Design review of the part built by this model. Coordinates are the model's own, in mm. Coordinates: 2 decimals unless noted, no trailing zeros. Loops run counter-clockwise (first coordinate to the right, second up) from the corner with the lowest first, then second, coordinate; pieces in that order, holes last.
Q1. Add section C-C on x = 29. Give the boundary of the cut face in (y, z), and give its area (3 significant figures).
Q2. Wall thickness on probe 1 along Y at (x, z) = (89, 3.15); probe 2 along Y at (x, z) = (94.5, 4.6); probe 3 along Y at (x, z) = (20, 1.6): over which ranges is each line inside the solid? List them lowest first.
Q3. For P1, Ø1.4, axis at y = -38, z = 3.5, coming from the +X side; P2, Ø2, axis at x = 10.5, z = 1.5, coming from the -Y side; P3, Ø3, axis at x = 85, z = 3.5, coming from the +Y side; P4, Ø2, axis at x = 28, y = -12.5, coming from the -Z side, all flat-tipped, find the tip position at first contact; note any pin that passes through.
Q4. Add section B-B on y = -24. Give the boundary of the cut face in (x, z).
Q5. Add section A-A on x = 94. Give the boundary of the cut face in (y, z).
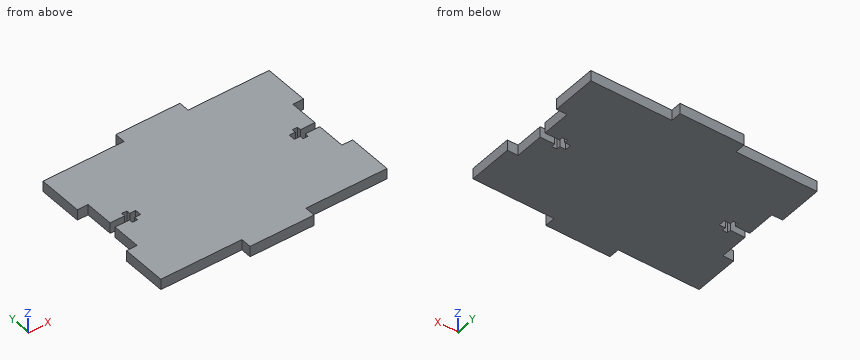
Autodesk Inventor part; units mm, degrees
ref_plane "工作平面2" through (-5, -77, -121) normal (-1, 0, 0) x (0, 0, 1)
ref_plane "工作平面3" through (101, -77, -121) normal (1, 0, 0) x (0, 1, 0)
ref_plane "YZ Plane" through (0, 0, 0) normal (1, 0, 0) x (0, 1, 0)
sketch "slot" plane through (0, 0, 0) normal (0, 0, 1) x (1, 0, 0)
  line L0 (-18.25, 14.2) -> (-11.75, 11.8) construction
  line L1 (-11.75, 14.2) -> (-18.25, 11.8) construction
  line L2 (-18.25, 14.2) -> (-16.5, 14.2)
  line L3 (-13.5, 14.2) -> (-11.75, 14.2)
  line L4 (-16.5, 9) -> (-16.5, 11.8)
  line L5 (-16.5, 14.2) -> (-16.5, 21)
  line L6 (-13.5, 21) -> (-13.5, 14.2)
  line L7 (-13.5, 11.8) -> (-13.5, 9)
  line L8 (-11.75, 11.8) -> (-13.5, 11.8)
  line L9 (-16.5, 11.8) -> (-18.25, 11.8)
  line L10 (-16.5, 21) -> (-13.5, 21)
  line L11 (-13.5, 9) -> (-16.5, 9)
  line L12 (-11.75, 14.2) -> (-11.75, 11.8)
  line L13 (-18.25, 11.8) -> (-18.25, 14.2)
  point P0 (-15, 21)
  point P1 (-15, 13)
  dimension "d8" = 3
  dimension "d9" = 12
  dimension "d10" = 6.5
  dimension "d11" = 2.4
  dimension "d12" = 8
ref_plane "工作平面1" through (0, 0, 0) normal (0, 0, 1) x (1, 0, 0)
sketch "草图2" plane through (0, 0, 0) normal (0, 0, 1) x (1, 0, 0)
  line L0 (74, -10) -> (74, -69)
  line L1 (74, -69) -> (69, -69)
  line L2 (69, -69) -> (69, -10)
  line L3 (69, -10) -> (74, -10)
  circle A0 centre (48, 2.5) radius 1.5
  circle A1 centre (48, -74.5) radius 1.5
  line L4 (33, -77) -> (33, -72)
  line L5 (63, -77) -> (33, -77)
  line L6 (63, -72) -> (63, -77)
  line L7 (96, -72) -> (63, -72)
  line L8 (96, 0) -> (96, -72)
  line L9 (63, 0) -> (96, 0)
  line L10 (63, 5) -> (63, 0)
  line L11 (33, 5) -> (63, 5)
  line L12 (33, 0) -> (33, 5)
  line L13 (0, 0) -> (33, 0)
  line L14 (0, -72) -> (0, 0)
  line L15 (33, -72) -> (0, -72)
extrude "拉伸2" add sketch "草图2" along normal blind 5 contours L0 L1 L2 L3 | A0 | A1 | L4 L15 L14 L13 L12 L11 L10 L9 L8 L7 L6 L5
sketch "草图3" plane through (0, -72, 0) normal (-1, 0, 0) x (0, 0, 1)
  line L0 (0, 0) -> (0, 72)
  line L1 (0, 0) -> (5, 0)
  line L2 (5, 72) -> (5, 0)
  line L3 (0, 72) -> (5, 72)
  circle A0 centre (2.5, 36) radius 1.5
  circle A1 centre (-35, -2.5) radius 1.5
  circle A2 centre (-85, -2.5) radius 1.5
  circle A3 centre (-85, 74.5) radius 1.5
  circle A4 centre (-35, 74.5) radius 1.5
  line L4 (-20, 0) -> (-20, -5)
  line L5 (0, 0) -> (-20, 0)
  line L6 (0, 21) -> (0, 0)
  line L7 (0, 21) -> (5, 21)
  line L8 (5, 21) -> (5, 51)
  line L9 (5, 51) -> (0, 51)
  line L10 (0, 72) -> (0, 51)
  line L11 (-20, 72) -> (0, 72)
  line L12 (-20, 77) -> (-20, 72)
  line L13 (-50, 77) -> (-20, 77)
  line L14 (-50, 72) -> (-50, 77)
  line L15 (-70, 72) -> (-50, 72)
  line L16 (-70, 77) -> (-70, 72)
  line L17 (-100, 77) -> (-70, 77)
  line L18 (-100, 72) -> (-100, 77)
  line L19 (-121, 72) -> (-100, 72)
  line L20 (-121, 0) -> (-121, 72)
  line L21 (-100, 0) -> (-121, 0)
  line L22 (-100, -5) -> (-100, 0)
  line L23 (-70, -5) -> (-100, -5)
  line L24 (-70, 0) -> (-70, -5)
  line L25 (-50, 0) -> (-70, 0)
  line L26 (-50, -5) -> (-50, 0)
  line L27 (-20, -5) -> (-50, -5)
ref_plane "工作平面2" through (-5, -77, -121) normal (-1, 0, 0) x (0, 0, 1)
extrude "拉伸3" add sketch "草图3" along normal up to surface (5 mm away) contours L0 L7 L2 L1 | L0 L3 L2 L9
sketch "草图4" plane through (96, -72, 0) normal (1, 0, 0) x (0, 0, -1)
  line L0 (0, 72) -> (0, 0)
  line L1 (0, 72) -> (-5, 72)
  line L2 (-5, 0) -> (-5, 72)
  line L3 (0, 0) -> (-5, 0)
  circle A0 centre (-2.5, 36) radius 1.5
  circle A1 centre (35, -2.5) radius 1.5
  circle A2 centre (85, -2.5) radius 1.5
  circle A3 centre (85, 74.5) radius 1.5
  circle A4 centre (35, 74.5) radius 1.5
  line L4 (20, 0) -> (20, -5)
  line L5 (20, -5) -> (50, -5)
  line L6 (50, -5) -> (50, 0)
  line L7 (50, 0) -> (70, 0)
  line L8 (70, 0) -> (70, -5)
  line L9 (70, -5) -> (100, -5)
  line L10 (100, -5) -> (100, 0)
  line L11 (100, 0) -> (121, 0)
  line L12 (121, 0) -> (121, 72)
  line L13 (121, 72) -> (100, 72)
  line L14 (100, 72) -> (100, 77)
  line L15 (100, 77) -> (70, 77)
  line L16 (70, 77) -> (70, 72)
  line L17 (70, 72) -> (50, 72)
  line L18 (50, 72) -> (50, 77)
  line L19 (50, 77) -> (20, 77)
  line L20 (20, 77) -> (20, 72)
  line L21 (20, 72) -> (0, 72)
  line L22 (0, 72) -> (0, 51)
  line L23 (0, 51) -> (-5, 51)
  line L24 (-5, 51) -> (-5, 21)
  line L25 (-5, 21) -> (0, 21)
  line L26 (0, 21) -> (0, 0)
  line L27 (0, 0) -> (20, 0)
ref_plane "工作平面3" through (101, -77, -121) normal (1, 0, 0) x (0, 1, 0)
extrude "拉伸4" add sketch "草图4" along normal up to surface (5 mm away) contours L0 L23 L2 L1 | L0 L3 L2 L25
sketch "草图5" plane through (0, 0, 5) normal (0, 0, 1) x (1, 0, 0)
  line L0 (0, -21) -> (0, -51)
  line L1 (96, -51) -> (96, -21)
  line L2 (-5, -37.5) -> (-5, -34.5)
  line L3 (101, -34.5) -> (101, -37.5)
  line L4 (6.8, -39.25) -> (9.2, -32.75) construction
  line L5 (6.8, -32.75) -> (9.2, -39.25) construction
  line L6 (6.8, -39.25) -> (6.8, -37.5)
  line L7 (6.8, -34.5) -> (6.8, -32.75)
  line L8 (12, -37.5) -> (9.2, -37.5)
  line L9 (6.8, -37.5) -> (0, -37.5)
  line L10 (0, -34.5) -> (6.8, -34.5)
  line L11 (9.2, -34.5) -> (12, -34.5)
  line L12 (9.2, -32.75) -> (9.2, -34.5)
  line L13 (9.2, -37.5) -> (9.2, -39.25)
  line L14 (0, -37.5) -> (0, -34.5)
  line L15 (12, -34.5) -> (12, -37.5)
  line L16 (6.8, -32.75) -> (9.2, -32.75)
  line L17 (9.2, -39.25) -> (6.8, -39.25)
  line L18 (89.2, -32.75) -> (86.8, -39.25) construction
  line L19 (89.2, -39.25) -> (86.8, -32.75) construction
  line L20 (89.2, -32.75) -> (89.2, -34.5)
  line L21 (89.2, -37.5) -> (89.2, -39.25)
  line L22 (84, -34.5) -> (86.8, -34.5)
  line L23 (89.2, -34.5) -> (96, -34.5)
  line L24 (96, -37.5) -> (89.2, -37.5)
  line L25 (86.8, -37.5) -> (84, -37.5)
  line L26 (86.8, -39.25) -> (86.8, -37.5)
  line L27 (86.8, -34.5) -> (86.8, -32.75)
  line L28 (96, -34.5) -> (96, -37.5)
  line L29 (84, -37.5) -> (84, -34.5)
  line L30 (89.2, -39.25) -> (86.8, -39.25)
  line L31 (86.8, -32.75) -> (89.2, -32.75)
  point P0 (0, 0)
extrude "拉伸5" cut sketch "草图5" against normal through all
properties part number "back"
Entries:
1. outline: (-72, 0) - (0, 0) - (0, 5) - (-72, 5) - close
1. area: 360 mm2
2. probe 1: y = -72 to -39.25, -32.75 to 0
2. probe 2: y = -72 to -37.5, -34.5 to 0
2. probe 3: y = -72 to 0
3. P1: stops at x = 96
3. P2: stops at y = -72
3. P3: stops at y = 0
3. P4: stops at z = 0
4. outline: (0, 0) - (96, 0) - (96, 5) - (0, 5) - close
5. outline: (-72, 0) - (-37.5, 0) - (-37.5, 5) - (-72, 5) - close; (-34.5, 0) - (0, 0) - (0, 5) - (-34.5, 5) - close
